Job drawing, mm, ordinate dimensions from the low corner. One solid piece. A direction names the side the tool comes from. Give positions to 0.01 mm unless a question says otherwise; leave off trailing zeros. Order: outer loops, then holes, each group sorted by start corner. A loop starts at its lowest first (then second) coordinate and runs counter-clockwise, first axis right, second up.
1. Which spindle directions (+Z, -Z, +X, -X, +Y, -Y) get a long thin tool onto all of the face, cutting with end or side? Do the marked faces 1, 2 and 3. Say none if no direction does.
2. Drop flat-ended pins along their axis: pin 1 Ø5.5 at (x, y) = (41, 4) entering from +Z; pin 2 Ø3.5 at (x, y) = (38.5, 8) entering from -Z; pin 3 Ø0.9 at (x, z) = (46, 37.5) entering from +Y. Give the stop position or say it passes through.
3. Slice it at B-B on y = 34.5. List the corners of the cut face in (x, z).
4. Probe line 1 (X direction, y = 8, z = 64); line 2 (Z direction, x = 42, y = 7.5); line 3 (X direction, y = 18, z = 33.5). List the from-to ranges inside material, lowest first.
5. Slice it at D-D on z = 17. List the corners of the cut face in (x, y).
6. Slice it at C-C on y = 12.5. List the corners of the cut face in (x, z), and give its area (3 significant figures).
7. Slice it at A-A on z = 54. List the corners of the cut face in (x, y), and give its area (3 significant figures).
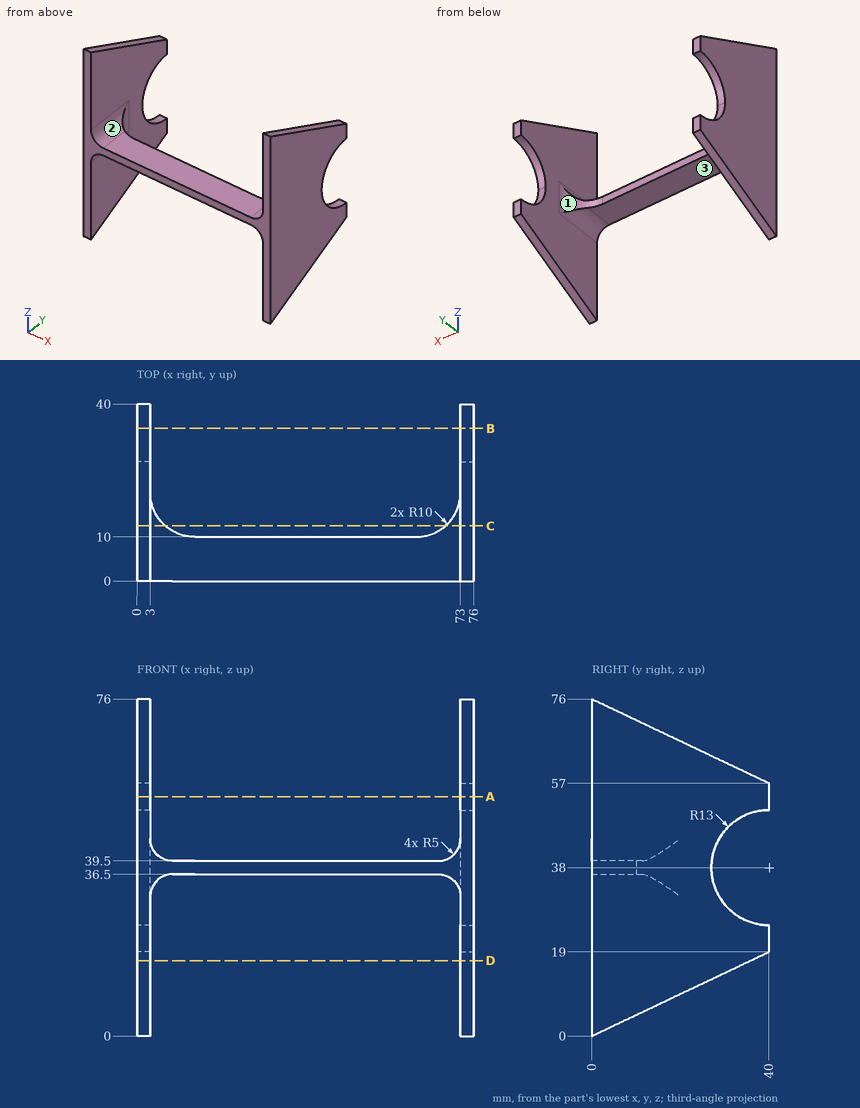
Data:
1. face 1: +Z, -Z, +Y
1. face 2: +Z, +Y, -Y
1. face 3: -Z, +Y, -Y
2. pin 1: stops at z = 39.5
2. pin 2: stops at z = 36.5
2. pin 3: stops at y = 10
3. outline: (0, 16.39) - (3, 16.39) - (3, 26.22) - (0, 26.22) - close; (0, 49.78) - (3, 49.78) - (3, 59.61) - (0, 59.61) - close; (73, 16.39) - (76, 16.39) - (76, 26.22) - (73, 26.22) - close; (73, 49.78) - (76, 49.78) - (76, 59.61) - (73, 59.61) - close
4. line 1: x = 0 to 3, 73 to 76
4. line 2: z = 36.5 to 39.5
4. line 3: x = 0 to 3.2, 72.8 to 76
5. outline: (0, 0) - (3, 0) - (3, 35.79) - (0, 35.79) - close; (73, 0) - (76, 0) - (76, 35.79) - (73, 35.79) - close
6. outline: (0, 5.94) - (3, 5.94) - (3, 31.5) arc R5 cw to (6.39, 36.23) - (6.39, 39.77) arc R5 cw to (3, 44.5) - (3, 70.06) - (0, 70.06) - close; (69.61, 36.23) arc R5 cw to (73, 31.5) - (73, 5.94) - (76, 5.94) - (76, 70.06) - (73, 70.06) - (73, 44.5) arc R5 cw to (69.61, 39.77) - close
6. area: 426 mm2
7. outline: (0, 0) - (3, 0) - (3, 40) - (0, 40) - close; (73, 0) - (76, 0) - (76, 40) - (73, 40) - close
7. area: 240 mm2
